```python
from build123d import *

# Parameters (mm, degrees)
SKETCH_1_R      = 3.6
EXTRUDE_1_DEPTH = 4


with BuildPart() as part:
    # Эскиз1 → Бобышка-Вытянуть1 (new body)
    with BuildSketch(Plane.XZ.offset(-165.322557711)):
        with BuildLine():
            Line((-231.421328736, -112.083155458), (-235.069374415, -113.356756687))
            ThreePointArc((-235.069374415, -113.356756687), (-237.498106164, -115.18254085), (-238.421328736, -118.077344091))
            Line((-238.421328736, -118.077344091), (-238.421328736, -130.787626703))
            ThreePointArc((-238.421328736, -130.787626703), (-236.316131977, -134.864404131), (-231.773283057, -135.508214107))
            Line((-231.773283057, -135.508214107), (-231.421328736, -135.385340246))
            Line((-231.421328736, -135.385340246), (-224.069374415, -132.81863498))
            ThreePointArc((-224.069374415, -132.81863498), (-219.526525495, -133.462444956), (-217.421328736, -137.539222384))
            Line((-217.421328736, -137.539222384), (-217.421328736, -158.195492647))
            ThreePointArc((-217.421328736, -158.195492647), (-218.88579483, -161.731026553), (-222.421328736, -163.195492647))
            Line((-222.421328736, -163.195492647), (-226.421328736, -163.195492647))
            ThreePointArc((-226.421328736, -163.195492647), (-229.956862642, -161.731026553), (-231.421328736, -158.195492647))
            Line((-231.421328736, -158.195492647), (-231.421328736, -157.255548243))
            ThreePointArc((-231.421328736, -157.255548243), (-233.526525495, -153.178770815), (-238.069374415, -152.534960839))
            Line((-238.069374415, -152.534960839), (-245.773283057, -155.224539965))
            ThreePointArc((-245.773283057, -155.224539965), (-250.316131977, -154.580729989), (-252.421328736, -150.503952561))
            Line((-252.421328736, -150.503952561), (-252.421328736, -108.136343856))
            ThreePointArc((-252.421328736, -108.136343856), (-251.498106164, -105.241540615), (-249.069374415, -103.415756451))
            Line((-249.069374415, -103.415756451), (-234.773283057, -98.424722589))
            ThreePointArc((-234.773283057, -98.424722589), (-232.344551308, -96.598938425), (-231.421328736, -93.704135185))
            Line((-231.421328736, -93.704135185), (-231.421328736, -22.195492647))
            ThreePointArc((-231.421328736, -22.195492647), (-229.956862642, -18.659958741), (-226.421328736, -17.195492647))
            Line((-226.421328736, -17.195492647), (-222.421328736, -17.195492647))
            ThreePointArc((-222.421328736, -17.195492647), (-218.88579483, -18.659958741), (-217.421328736, -22.195492647))
            Line((-217.421328736, -22.195492647), (-217.421328736, -103.64513542))
            ThreePointArc((-217.421328736, -103.64513542), (-218.344551308, -106.539938661), (-220.773283057, -108.365722824))
            Line((-220.773283057, -108.365722824), (-231.421328736, -112.083155458))
        make_face()
        with Locations((-224.421328736, -68.195492647)):
            Circle(SKETCH_1_R, mode=Mode.SUBTRACT)
        with BuildLine():
            Line((-228.021328736, -139.195492647), (-228.021328736, -155.195492647))
            ThreePointArc((-228.021328736, -155.195492647), (-224.421328736, -158.795492647), (-220.821328736, -155.195492647))
            Line((-220.821328736, -155.195492647), (-220.821328736, -139.195492647))
            ThreePointArc((-220.821328736, -139.195492647), (-224.421328736, -135.595492647), (-228.021328736, -139.195492647))
        make_face(mode=Mode.SUBTRACT)
        with BuildLine():
            Line((-228.021328736, -24.195492647), (-228.021328736, -32.195492647))
            ThreePointArc((-228.021328736, -32.195492647), (-224.421328736, -35.795492647), (-220.821328736, -32.195492647))
            Line((-220.821328736, -32.195492647), (-220.821328736, -24.195492647))
            ThreePointArc((-220.821328736, -24.195492647), (-224.421328736, -20.595492647), (-228.021328736, -24.195492647))
        make_face(mode=Mode.SUBTRACT)
    extrude(amount=EXTRUDE_1_DEPTH)


solid = part.part
```
For this review, take the finished solid that the model builds, in its own axes (mm). A direction names the side the tool comes from. Give positions to 0.01 mm unless a question says otherwise; leave off trailing zeros. Write each loop counter-clockwise with the first axis right and the second up, starting at its lowest first coordinate (ties: lowest second). Pieces come first, ordered by that corner, then holes. Notation, with made-up numbers: M 33.5,62.5 L 66.5,62.5 A28 ccw 66.5,95.5 Z; hole C 49.5,52 d10. An arc over 180 degrees is marked long. Answer as CSV lines item,"result".
1. For faces 1 (the cylindrical face through (-224.5, 163.351, -158.795)), 2 (the cylindrical face through (-232.37, 163.351, -96.634)), list the 3-axis set-ups (+Z, -Z, +X, -X, +Y, -Y) from which the entire face can be reached by the end or side of a thin tool; tool diameter is ignored.
Findings:
face 1,"+Y, -Y"
face 2,"+Z, -X, +Y, -Y"
2. Consider section B-B, the plane y = 162.75. Count the separate pieces of the cut face and the enclosed holes in it, then the cut area to 3 significant figures.
Findings:
separate pieces,"1"
enclosed holes,"3"
area,"2,350 mm2"
3. Consider section A-A, the plane z = -84.5. Write out the cut boundary in (x, y), then the cut area to 3 significant figures.
Findings:
outline,"M -231.42,161.32 L -217.42,161.32 L -217.42,165.32 L -231.42,165.32 Z"
area,"56.0 mm2"
4. For pin 1 (2 mm diameter, centred on y = 163, z = -29, fed in from -X); pin 2 (1 mm diameter, centred on x = -233, z = -49, fed in from +Y); pin 3 (1 mm diameter, centred on x = -235.5, y = 163.5, fed in from -Z); pin 4 (1.2 mm diameter, centred on y = 162.5, z = -127.5, fed in from +X), all flat-tipped, find the tip position at first contact; note any pin that passes through.
Findings:
pin 1,"stops at x = -231.42"
pin 2,"passes through"
pin 3,"stops at z = -152.46"
pin 4,"stops at x = -238.42"
5. Draft analysis for pull direction X (two halves, no side actions). For faces 3 (the cylindrical face through (-236.37, 163.351, -134.825)), 4 (the flat face through (-217.421, 163, -62)), 5 (the cylindrical face through (-251.523, 163.351, -105.277)), state which applies: +X half, -X half, draft (parallel to the pull), parting line (faces both ways), or undercut.
Findings:
face 3,"undercut"
face 4,"+X half"
face 5,"-X half"
6. Consider section C-C, the plane x = -241. Write out the cut boundary in (y, z).
Findings:
outline,"M 161.32,-153.56 L 165.32,-153.56 L 165.32,-100.6 L 161.32,-100.6 Z"
7. Wall thickness on line 1 (Z direction, x = -227, y = 163.1); line 2 (X direction, y = 161.65, z = -148); line 3 (Z direction, x = -222.5, y = 162.4): over which ranges is each line inside the solid? List them lowest first.
Findings:
line 1,"z = -163.16 to -157.71, -136.68 to -133.84, -110.54 to -70.71, -65.68 to -34.71, -21.68 to -17.23"
line 2,"x = -252.42 to -228.02, -220.82 to -217.42"
line 3,"z = -163.2 to -158.24, -136.15 to -132.54, -108.97 to -71.24, -65.15 to -35.24, -21.15 to -17.2"
